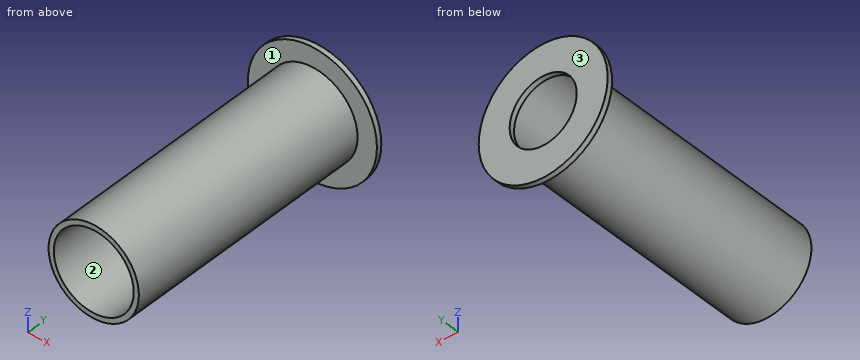
```python
from build123d import *

# Parameters (mm, degrees)
SKETCH1_R           = 7
SKETCH1_R_2         = 6.2
BOSS_EXTRUDE1_DEPTH = 20
SKETCH4_R           = 10
SKETCH4_R_2         = 5.2
BOSS_EXTRUDE3_DEPTH = 0.8


with BuildPart() as part:
    # Sketch1 → Boss-Extrude1 (new body, symmetric)
    with BuildSketch(Plane(origin=(0, 0, 0), x_dir=(1, 0, 0), z_dir=(0, 1, 0))):
        Circle(SKETCH1_R)
        Circle(SKETCH1_R_2, mode=Mode.SUBTRACT)
    extrude(amount=BOSS_EXTRUDE1_DEPTH, both=True)

    # Sketch4 → Boss-Extrude3 (add)
    with BuildSketch(Plane(origin=(0, 20, 0), x_dir=(1, 0, 0), z_dir=(0, 1, 0))):
        Circle(SKETCH4_R)
        Circle(SKETCH4_R_2, mode=Mode.SUBTRACT)
    extrude(amount=BOSS_EXTRUDE3_DEPTH)


solid = part.part
```
Part model, mm, in its own coordinate system. Face numbers are marked on the shaded views. Round coordinates to 2 decimals unless told otherwise and drop trailing zeros. Write each loop counter-clockwise with the first axis right and the second up, starting at its lowest first coordinate (ties: lowest second). Pieces come first, ordered by that corner, then holes. Notation, with made-up numbers: (57, 7) -> (78, 7) arc R25 cw to (78, 44) -> close; hole circle Ø2 at (59, 76.25). An arc over 180 degrees is marked (long way). Return JSON: item names as keys, results as strings. Group by question number.
Q1. Probe L1, parallel to X at y = -6.5, z = 0; L2, parallel to Z at x = 0, y = 20.35. List the from-to ranges inside material, lowest first. Write a range as [from, to].
Q2. Pin check, flat tips, straight feed: pin 1 (10 mm diameter, centred on x = -7.5, z = 7.5, fed in from -Y); pin 2 (6 mm diameter, centred on x = 6, y = 1, fed in from -Z); pin 3 (8 mm diameter, centred on x = -6, y = 14.5, fed in from -Z); pin 4 (6 mm diameter, centred on y = 2, z = -2, fed in from -X). Stop position of each tip, or through.
Q3. Saw through at A-A on z = 0. Write the cut outline in (x, y), plus the area to 3 significant figures.
Q4. Saw through at D-D on z = 5.75. Write the cut outline in (x, y).
Q5. Saw through at B-B on x = 0. Write the cut outline in (y, z).
Q6. Saw through at C-C on y = -12. Write the cut outline in (x, z), plus the area to 3 significant figures.
Q7. Mould opens along Y. For the marked faces 1, 2 and 3 say: pulls with the +Y half, pulls with the -Y half, needs draft (parallel to the pull), parting line crosses it, or undercut.
Answer:
{
 "1": {"L1": "[-7, -6.2], [6.2, 7]", "L2": "[-10, -5.2], [5.2, 10]"},
 "2": {"pin 1": "y = -20", "pin 2": "z = -6.32", "pin 3": "z = -6.71", "pin 4": "x = -7"},
 "3": {"outline": "(-10, 20) -> (-7, 20) -> (-7, -20) -> (-6.2, -20) -> (-6.2, 20) -> (-5.2, 20) -> (-5.2, 20.8) -> (-10, 20.8) -> close; (5.2, 20) -> (6.2, 20) -> (6.2, -20) -> (7, -20) -> (7, 20) -> (10, 20) -> (10, 20.8) -> (5.2, 20.8) -> close", "area": "71.7 mm2"},
 "4": {"outline": "(-8.18, 20) -> (-3.99, 20) -> (-3.99, -20) -> (-2.32, -20) -> (-2.32, 20) -> (2.32, 20) -> (2.32, -20) -> (3.99, -20) -> (3.99, 20) -> (8.18, 20) -> (8.18, 20.8) -> (-8.18, 20.8) -> close"},
 "5": {"outline": "(-20, -7) -> (20, -7) -> (20, -10) -> (20.8, -10) -> (20.8, -5.2) -> (20, -5.2) -> (20, -6.2) -> (-20, -6.2) -> close; (-20, 6.2) -> (20, 6.2) -> (20, 5.2) -> (20.8, 5.2) -> (20.8, 10) -> (20, 10) -> (20, 7) -> (-20, 7) -> close"},
 "6": {"outline": "circle Ø14 at (0, 0); hole circle Ø12.4 at (0, 0)", "area": "33.2 mm2"},
 "7": {"face 1": "pulls with the -Y half", "face 2": "needs draft", "face 3": "pulls with the +Y half"}
}
